from build123d import *

# Parameters (mm, degrees)
CROQUIS1_W             = 37.5
CROQUIS1_H             = 30
BRIDA_BASE1_DEPTH      = 2
BRIDA_DE_ARISTA1_DEPTH = 30
CROQUIS9_R             = 1.5
CORTAR_EXTRUIR1_DEPTH  = 10
REDONDEO1_R            = 5
CROQUIS10_R            = 6.466120371
CROQUIS10_R_2          = 1
CORTAR_EXTRUIR2_DEPTH  = 2
REDONDEO2_R            = 5


# Sheet-metal steps are written as plain solids
with BuildPart() as part:
    # Croquis1 → Brida base1 (new body)
    with BuildSketch(Plane(origin=(0, 0, 0), x_dir=(1, 0, 0), z_dir=(0, 1, 0))):
        Rectangle(CROQUIS1_W, CROQUIS1_H)
    extrude(amount=-BRIDA_BASE1_DEPTH)

    # Brida de arista1 section (across the edge) → Brida de arista1 (add)
    with BuildSketch(Plane(origin=(-19.25, 0, -15), x_dir=(1, 0, 0), z_dir=(0, 0, 1))):
        with BuildLine():
            Line((-2, 0.5), (-2, 42.5))
            Line((-2, 42.5), (0, 42.5))
            Line((0, 42.5), (0, 0.5))
            ThreePointArc((0, 0.5), (0.146446609, 0.146446609), (0.5, 0))
            Line((0.5, 0), (0.5, -2))
            ThreePointArc((0.5, -2), (-1.267766953, -1.267766953), (-2, 0.5))
        make_face()
    extrude(amount=BRIDA_DE_ARISTA1_DEPTH)

    # Croquis9 → Cortar-Extruir1 (cut)
    with BuildSketch(Plane.XZ.offset(2)):
        with Locations(Location((-12.75, 5, 0), (0, 0, 270))):
            Circle(CROQUIS9_R)
        with Locations(Location((12.25, 5, 0), (0, 0, 270))):
            Circle(CROQUIS9_R)
        with Locations(Location((12.25, -5, 0), (0, 0, 270))):
            Circle(CROQUIS9_R)
        with Locations(Location((-12.75, -5, 0), (0, 0, 270))):
            Circle(CROQUIS9_R)
    extrude(amount=-CORTAR_EXTRUIR1_DEPTH, mode=Mode.SUBTRACT)

    # Redondeo1
    redondeo1_edges = [part.edges().sort_by_distance(p)[0] for p in [
        (18.75, -1, 15),
        (18.75, -1, -15),
    ]]
    fillet(redondeo1_edges, radius=REDONDEO1_R)

    # Croquis10 → Cortar-Extruir2 (cut)
    with BuildSketch(Plane.ZY.offset(21.25)):
        with Locations(Location((0, 26, 0), (0, 0, 270))):
            Circle(CROQUIS10_R)
        with Locations(Location((-12, 38, 0), (0, 0, 270))):
            Circle(CROQUIS10_R_2)
        with Locations(Location((12, 38, 0), (0, 0, 270))):
            Circle(CROQUIS10_R_2)
        with Locations(Location((12, 14, 0), (0, 0, 270))):
            Circle(CROQUIS10_R_2)
        with Locations(Location((-12, 14, 0), (0, 0, 270))):
            Circle(CROQUIS10_R_2)
    extrude(amount=-CORTAR_EXTRUIR2_DEPTH, mode=Mode.SUBTRACT)

    # Redondeo2
    redondeo2_edges = [part.edges().sort_by_distance(p)[0] for p in [
        (-20.25, 42.5, -15),
        (-20.25, 42.5, 15),
    ]]
    fillet(redondeo2_edges, radius=REDONDEO2_R)


solid = part.part
For this review, take the finished solid that the model builds, in its own axes (mm). Round coordinates to 2 decimals unless told otherwise and drop trailing zeros. Write each loop counter-clockwise with the first axis right and the second up, starting at its lowest first coordinate (ties: lowest second). Pieces come first, ordered by that corner, then holes. Notation, with made-up numbers: (64, 51.25) - (102, 51.25) arc R18 cw to (102, 76.25) - close; hole circle Ø4 at (33.5, -37). An arc over 180 degrees is marked (long way). Use a Markdown table: item, result.
Q1. We need section C-C (y = 29). Give the boundary of the cut face in (x, z).
Derived:
| item | result |
|---|---|
| outline | (-21.25, -15) - (-19.25, -15) - (-19.25, -5.73) - (-21.25, -5.73) - close; (-21.25, 5.73) - (-19.25, 5.73) - (-19.25, 15) - (-21.25, 15) - close |
Q2. We need section A-A (x = 12.25). Give the boundary of the cut face in (y, z), plus the area to 3 significant figures.
Derived:
| item | result |
|---|---|
| outline | (-2, -15) - (0, -15) - (0, -6.5) - (-2, -6.5) - close; (-2, -3.5) - (0, -3.5) - (0, 3.5) - (-2, 3.5) - close; (-2, 6.5) - (0, 6.5) - (0, 15) - (-2, 15) - close |
| area | 48.0 mm2 |
Q3. We need section B-B (z = -4.75). Give the boundary of the cut face in (x, y), plus the area to 3 significant figures.
Derived:
| item | result |
|---|---|
| outline | (-21.25, 0.5) arc R2.5 ccw to (-18.75, -2) - (-14.23, -2) - (-14.23, 0) - (-18.75, 0) arc R0.5 cw to (-19.25, 0.5) - (-19.25, 21.61) - (-21.25, 21.61) - close; (-21.25, 30.39) - (-19.25, 30.39) - (-19.25, 42.5) - (-21.25, 42.5) - close; (-11.27, -2) - (10.77, -2) - (10.77, 0) - (-11.27, 0) - close; (13.73, -2) - (18.75, -2) - (18.75, 0) - (13.73, 0) - close |
| area | 134 mm2 |
Q4. We need section D-D (z = -12). Give the boundary of the cut face in (x, y).
Derived:
| item | result |
|---|---|
| outline | (-21.25, 0.5) arc R2.5 ccw to (-18.75, -2) - (18.33, -2) - (18.33, 0) - (-18.75, 0) arc R0.5 cw to (-19.25, 0.5) - (-19.25, 13) - (-21.25, 13) - close; (-21.25, 15) - (-19.25, 15) - (-19.25, 37) - (-21.25, 37) - close; (-21.25, 39) - (-19.25, 39) - (-19.25, 42.08) - (-21.25, 42.08) - close |
Q5. Wall thickness on line 1 along Z through (x, y) = (-20, 26); line 2 along Z through (x, y) = (-20.45, 14); line 3 along X through (y, z) = (15, 1): over which ranges is each line inside the solid? List them lowest first.
Derived:
| item | result |
|---|---|
| line 1 | z = -15 to -6.47, 6.47 to 15 |
| line 2 | z = -15 to -13, -11 to 11, 13 to 15 |
| line 3 | x = -21.25 to -19.25 |
Q6. Clearance check with flat-ended pins moving along their axes: pin 1 (15 mm diameter, centred on x = 7.5, z = -3.5, fed in from +Y); pin 2 (3 mm diameter, centred on y = 38, z = 12, fed in from -X); pin 3 (4 mm diameter, centred on y = 20.5, z = 10, fed in from +X). State where each tip first meets the part, or that it passes through.
Derived:
| item | result |
|---|---|
| pin 1 | stops at y = 0 |
| pin 2 | stops at x = -21.25 |
| pin 3 | stops at x = -19.25 |
Q7. The part is to be moulded in two halves that separate along Y. For faces 1 (the cylindrical face through (12.3, -1, 6.5)), 2 (the cylindrical face through (-20, 13, 12)), 3 (the flat face through (0, 0, 0)), say which applies: pulls with the +Y half, pulls with the -Y half, needs draft (parallel to the pull), parting line crosses it, or undercut.
Derived:
| item | result |
|---|---|
| face 1 | needs draft |
| face 2 | undercut |
| face 3 | pulls with the +Y half |
